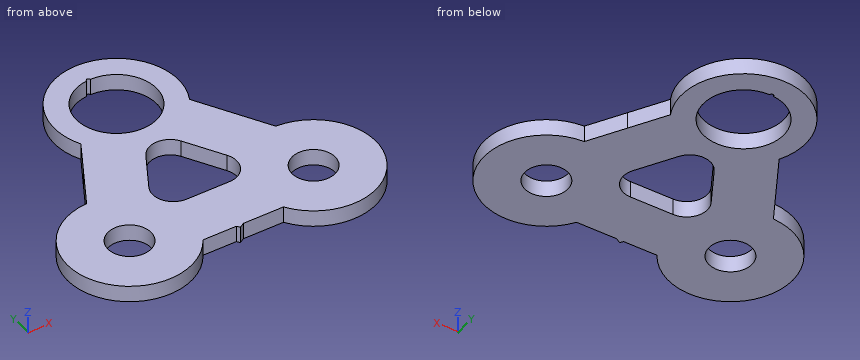
from build123d import *

# Parameters (mm, degrees)
SKETCH_1_R          = 5.2
EXTRUDE_1_DEPTH     = 4
CUT_EXTRUDE_1_DEPTH = 4


with BuildPart() as part:
    # 草图1 → 凸台-拉伸1 (new body)
    with BuildSketch(Plane.XY):
        with BuildLine():
            Line((-18.494622549, 4.742999843), (-23.409453688, -3.769737399))
            ThreePointArc((-23.409453688, -3.769737399), (-35.781809628, -26.257000157), (-10.121090849, -26.785856986))
            Line((-10.121090849, -26.785856986), (-1.94731163, -26.785856986))
            Line((-1.94731163, -26.785856986), (-1.47982289, -27.531216606))
            Line((-1.47982289, -27.531216606), (-0.291428571, -26.785856986))
            Line((-0.291428571, -26.785856986), (9.538233706, -26.785856986))
            ThreePointArc((9.538233706, -26.785856986), (35.198952485, -26.257000157), (22.826596545, -3.769737399))
            Line((22.826596545, -3.769737399), (17.911765406, 4.742999843))
            Line((17.911765406, 4.742999843), (12.996934268, 13.255737086))
            ThreePointArc((12.996934268, 13.255737086), (-0.291428571, 35.214143014), (-13.579791411, 13.255737086))
            Line((-13.579791411, 13.255737086), (-18.494622549, 4.742999843))
        make_face()
        with Locations((-0.291428571, 20.214143014)):
            Circle(SKETCH_1_R, mode=Mode.SUBTRACT)
        with Locations((22.208571429, -18.757000157)):
            Circle(SKETCH_1_R, mode=Mode.SUBTRACT)
        with Locations((-22.791428571, -18.757000157)):
            Circle(SKETCH_1_R, mode=Mode.SUBTRACT)
        with BuildLine():
            Line((9.268171867, -6.285856986), (4.038698447, 2.771856673))
            ThreePointArc((4.038698447, 2.771856673), (-0.291428571, 5.271856673), (-4.62155559, 2.771856673))
            Line((-4.62155559, 2.771856673), (-9.85102901, -6.285856986))
            ThreePointArc((-9.85102901, -6.285856986), (-9.85102901, -11.285856986), (-5.520901991, -13.785856986))
            Line((-5.520901991, -13.785856986), (4.938044848, -13.785856986))
            ThreePointArc((4.938044848, -13.785856986), (9.268171867, -11.285856986), (9.268171867, -6.285856986))
        make_face(mode=Mode.SUBTRACT)
    extrude(amount=EXTRUDE_1_DEPTH)

    # 草图2 → 切除-拉伸1 (cut)
    with BuildSketch(Plane.XY.offset(4)):
        with BuildLine():
            ThreePointArc((-0.291428571, 29.914143014), (-0.77677081, 30.355150727), (-1.217778524, 29.869808489))
            ThreePointArc((-1.217778524, 29.869808489), (0.172276557, 10.525232985), (-0.291428571, 29.914143014))
        make_face()
    extrude(amount=-CUT_EXTRUDE_1_DEPTH, mode=Mode.SUBTRACT)


solid = part.part
Check sheet for the modelled part. Datum: model origin and axes. Units: mm. Round coordinates to 2 decimals unless told otherwise and drop trailing zeros. Order: outer loops, then holes, each group sorted by start corner. A loop starts at its lowest first (then second) coordinate and runs counter-clockwise, first axis right, second up.
(1) Go/stop test with flat-tipped pins: P1, Ø1, axis at y = 2.5, z = 2, coming from the -X side; P2, Ø1.2, axis at x = 3, z = 2, coming from the -Y side; P3, Ø1.5, axis at y = -15, z = 1.5, coming from the +X side. Record where each tip stops, or that it passes through.
(2) Cross-section at D-D, the plane y = -25. Enter the section's corners in (x, z).
(3) Cross-section at A-A, the plane y = 16. Enter the section's corners in (x, z), and give its area (3 significant figures).
(4) Cross-section at C-C, the plane y = -11.5. Enter the section's corners in (x, z).
(5) Cross-section at B-B, the plane z = 0.75. Enter the section's corners in (x, y).
(6) Scan lines: probe 1 along X at (y, z) = (-19, 0.9); probe 2 along Y at (x, z) = (-7, 1.55); probe 3 along Y at (x, z) = (4, 1.85). Record each from-to range of solid material in increasing order.
Check sheet entries:
1. P1: stops at x = -20.08
1. P2: stops at y = -26.79
1. P3: stops at x = 36.9
2. outline: (-36.43, 0) - (35.85, 0) - (35.85, 4) - (-36.43, 4) - close
3. outline: (-14.69, 0) - (-9.03, 0) - (-9.03, 4) - (-14.69, 4) - close; (8.45, 0) - (14.1, 0) - (14.1, 4) - (8.45, 4) - close
3. area: 45.3 mm2
4. outline: (-35.92, 0) - (-9.72, 0) - (-9.72, 4) - (-35.92, 4) - close; (9.14, 0) - (35.34, 0) - (35.34, 4) - (9.14, 4) - close
5. outline: (-23.41, -3.77) arc R15 ccw (long way) to (-10.12, -26.79) - (-1.95, -26.79) - (-1.48, -27.53) - (-0.29, -26.79) - (9.54, -26.79) arc R15 ccw (long way) to (22.83, -3.77) - (13, 13.26) arc R15 ccw (long way) to (-13.58, 13.26) - close; hole circle Ø10.4 at (-22.79, -18.76); hole (-9.85, -6.29) arc R5 ccw to (-5.52, -13.79) - (4.94, -13.79) arc R5 ccw to (9.27, -6.29) - (4.04, 2.77) arc R5 ccw to (-4.62, 2.77) - close; hole (-1.22, 29.87) arc R9.7 ccw (long way) to (-0.29, 29.91) arc R0.46 ccw to start; hole circle Ø10.4 at (22.21, -18.76)
6. probe 1: x = -37.79 to -27.99, -17.6 to 17.01, 27.4 to 37.21
6. probe 2: y = -26.79 to -13.56, -1.35 to 13.21, 27.22 to 33.63
6. probe 3: y = -26.79 to -13.79, 2.84 to 11.52, 28.91 to 34.59
